Geometry check sheet. Reference: the model listing, model coordinates, mm. Round coordinates to 2 decimals unless told otherwise and drop trailing zeros. Order: outer loops, then holes, each group sorted by start corner. A loop starts at its lowest first (then second) coordinate and runs counter-clockwise, first axis right, second up. Notation, with made-up numbers: (-27.5, 39.25) - (16.5, 39.25) arc R9 ccw to (16.5, 43.25) - close; hole circle Ø8 at (86, 4). An arc over 180 degrees is marked (long way). Return JSON: item names as keys, results as strings. Group by question number.
Q1. Sectioned sample at C-C, the plane z = -10.5. Record the cut outline in (x, y).
Q2. Sectioned sample at A-A, the plane x = 5. Record the cut outline in (y, z).
Q3. Sectioned sample at D-D, the plane z = -18. Record the cut outline in (x, y).
Q4. Sectioned sample at B-B, the plane z = 0. Record the cut outline in (x, y).
Q5. Material ranges on line 1 along X through (y, z) = (1.5, 0); line 2 along X through (y, z) = (2.1, -2); line 3 along Z through (x, y) = (34, 2.3), recorded low to high.
Q6. Gauge pin test, flat ends, axial feed: pin 1 Ø3.5 at (x, z) = (0.52, -4.74) entering from -Y; pin 2 Ø1.5 at (y, z) = (2, -8.5) entering from +X; pin 3 Ø1.5 at (x, y) = (29.5, 1) entering from -Z; pin 4 Ø1.5 at (x, y) = (42, 2) entering from +Z. Record the tip position at first contact, or that the pin passes through.
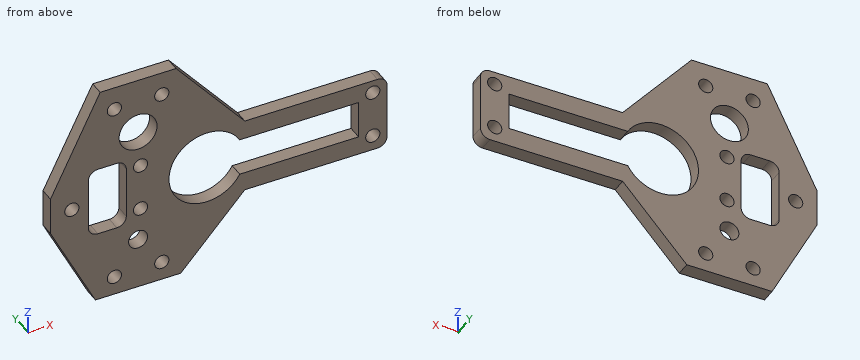
```python
from build123d import *

# Parameters (mm, degrees)
BASE_FLANGE1_DEPTH = 3
CUT_EXTRUDE1_REACH = 60.356
CUT_EXTRUDE2_REACH = 60.356
SKETCH3_R          = 1.5
SKETCH3_W          = 8
SKETCH3_H          = 15
CUT_EXTRUDE3_REACH = 60.356
SKETCH4_R          = 1.5
CUT_EXTRUDE4_REACH = 60.356
SKETCH5_R          = 2
SKETCH5_R_2        = 4
FILLET1_R          = 2


# Sheet-metal steps are written as plain solids
with BuildPart() as part:
    # Sketch1 → Base-Flange1 (new body)
    with BuildSketch(Plane(origin=(0, 0, 0), x_dir=(1, 0, 0), z_dir=(0, 1, 0))):
        Polygon((-18.480295105, -4), (-18.480295105, 4), (-9, 22.738303144), (9, 22.738303144), (22.519704895, 8), (52.519704895, 8), (52.519704895, -8), (22.519704895, -8), (8, -25.261696856), (-8, -25.261696856), align=None)
    extrude(amount=BASE_FLANGE1_DEPTH)

    # Sketch2 → Cut-Extrude1 (cut, up to next)
    with BuildSketch(Plane(origin=(0, 3, 0), x_dir=(1, 0, 0), z_dir=(0, 1, 0)), mode=Mode.PRIVATE) as cut_extrude1_sk1:
        with BuildLine():
            Line((21.447908125, 4), (46.519704895, 4))
            Line((46.519704895, 4), (46.519704895, -4))
            Line((46.519704895, -4), (21.447908125, -4))
            ThreePointArc((21.447908125, -4), (6.519704895, 0), (21.447908125, 4))
        make_face()
    cut_extrude1_tool1 = extrude(cut_extrude1_sk1.sketch, amount=-CUT_EXTRUDE1_REACH, mode=Mode.PRIVATE) & part.part
    add(cut_extrude1_tool1.solids().sort_by_distance((24.274518, 3, 0))[0], mode=Mode.SUBTRACT)

    # Sketch3 → Cut-Extrude2 (cut, up to next)
    with BuildSketch(Plane(origin=(0, 3, 0), x_dir=(1, 0, 0), z_dir=(0, 1, 0)), mode=Mode.PRIVATE) as cut_extrude2_sk1:
        with Locations(Location((-13.980295105, 0, 0), (0, 0, 270))):
            Circle(SKETCH3_R)
    cut_extrude2_tool1 = extrude(cut_extrude2_sk1.sketch, amount=-CUT_EXTRUDE2_REACH, mode=Mode.PRIVATE) & part.part
    # Sketch3 → Cut-Extrude2 (cut, up to next)
    with BuildSketch(Plane(origin=(0, 3, 0), x_dir=(1, 0, 0), z_dir=(0, 1, 0)), mode=Mode.PRIVATE) as cut_extrude2_sk2:
        with Locations((-6.480295105, 0)):
            Rectangle(SKETCH3_W, SKETCH3_H)
    cut_extrude2_tool2 = extrude(cut_extrude2_sk2.sketch, amount=-CUT_EXTRUDE2_REACH, mode=Mode.PRIVATE) & part.part
    add(cut_extrude2_tool1.solids().sort_by_distance((-13.980295, 3, 0))[0], mode=Mode.SUBTRACT)
    add(cut_extrude2_tool2.solids().sort_by_distance((-6.480295, 3, 0))[0], mode=Mode.SUBTRACT)

    # Sketch4 → Cut-Extrude3 (cut, up to next)
    with BuildSketch(Plane(origin=(0, 3, 0), x_dir=(1, 0, 0), z_dir=(0, 1, 0)), mode=Mode.PRIVATE) as cut_extrude3_sk1:
        with Locations(Location((-5, 18.738303144, 0), (0, 0, 270))):
            Circle(SKETCH4_R)
    cut_extrude3_tool1 = extrude(cut_extrude3_sk1.sketch, amount=-CUT_EXTRUDE3_REACH, mode=Mode.PRIVATE) & part.part
    # Sketch4 → Cut-Extrude3 (cut, up to next)
    with BuildSketch(Plane(origin=(0, 3, 0), x_dir=(1, 0, 0), z_dir=(0, 1, 0)), mode=Mode.PRIVATE) as cut_extrude3_sk2:
        with Locations(Location((5, 18.738303144, 0), (0, 0, 270))):
            Circle(SKETCH4_R)
    cut_extrude3_tool2 = extrude(cut_extrude3_sk2.sketch, amount=-CUT_EXTRUDE3_REACH, mode=Mode.PRIVATE) & part.part
    # Sketch4 → Cut-Extrude3 (cut, up to next)
    with BuildSketch(Plane(origin=(0, 3, 0), x_dir=(1, 0, 0), z_dir=(0, 1, 0)), mode=Mode.PRIVATE) as cut_extrude3_sk3:
        with Locations(Location((0.519704895, 4.738303144, 0), (0, 0, 270))):
            Circle(SKETCH4_R)
    cut_extrude3_tool3 = extrude(cut_extrude3_sk3.sketch, amount=-CUT_EXTRUDE3_REACH, mode=Mode.PRIVATE) & part.part
    # Sketch4 → Cut-Extrude3 (cut, up to next)
    with BuildSketch(Plane(origin=(0, 3, 0), x_dir=(1, 0, 0), z_dir=(0, 1, 0)), mode=Mode.PRIVATE) as cut_extrude3_sk4:
        with Locations(Location((-5, -20.261696856, 0), (0, 0, 270))):
            Circle(SKETCH4_R)
    cut_extrude3_tool4 = extrude(cut_extrude3_sk4.sketch, amount=-CUT_EXTRUDE3_REACH, mode=Mode.PRIVATE) & part.part
    # Sketch4 → Cut-Extrude3 (cut, up to next)
    with BuildSketch(Plane(origin=(0, 3, 0), x_dir=(1, 0, 0), z_dir=(0, 1, 0)), mode=Mode.PRIVATE) as cut_extrude3_sk5:
        with Locations(Location((5, -20.261696856, 0), (0, 0, 270))):
            Circle(SKETCH4_R)
    cut_extrude3_tool5 = extrude(cut_extrude3_sk5.sketch, amount=-CUT_EXTRUDE3_REACH, mode=Mode.PRIVATE) & part.part
    # Sketch4 → Cut-Extrude3 (cut, up to next)
    with BuildSketch(Plane(origin=(0, 3, 0), x_dir=(1, 0, 0), z_dir=(0, 1, 0)), mode=Mode.PRIVATE) as cut_extrude3_sk6:
        with Locations(Location((0.519704895, -5.261696856, 0), (0, 0, 270))):
            Circle(SKETCH4_R)
    cut_extrude3_tool6 = extrude(cut_extrude3_sk6.sketch, amount=-CUT_EXTRUDE3_REACH, mode=Mode.PRIVATE) & part.part
    # Sketch4 → Cut-Extrude3 (cut, up to next)
    with BuildSketch(Plane(origin=(0, 3, 0), x_dir=(1, 0, 0), z_dir=(0, 1, 0)), mode=Mode.PRIVATE) as cut_extrude3_sk7:
        with Locations(Location((49.519704895, 4.738303144, 0), (0, 0, 270))):
            Circle(SKETCH4_R)
    cut_extrude3_tool7 = extrude(cut_extrude3_sk7.sketch, amount=-CUT_EXTRUDE3_REACH, mode=Mode.PRIVATE) & part.part
    # Sketch4 → Cut-Extrude3 (cut, up to next)
    with BuildSketch(Plane(origin=(0, 3, 0), x_dir=(1, 0, 0), z_dir=(0, 1, 0)), mode=Mode.PRIVATE) as cut_extrude3_sk8:
        with Locations(Location((49.519704895, -5.261696856, 0), (0, 0, 270))):
            Circle(SKETCH4_R)
    cut_extrude3_tool8 = extrude(cut_extrude3_sk8.sketch, amount=-CUT_EXTRUDE3_REACH, mode=Mode.PRIVATE) & part.part
    add(cut_extrude3_tool1.solids().sort_by_distance((-5, 3, -18.738303))[0], mode=Mode.SUBTRACT)
    add(cut_extrude3_tool2.solids().sort_by_distance((5, 3, -18.738303))[0], mode=Mode.SUBTRACT)
    add(cut_extrude3_tool3.solids().sort_by_distance((0.519705, 3, -4.738303))[0], mode=Mode.SUBTRACT)
    add(cut_extrude3_tool4.solids().sort_by_distance((-5, 3, 20.261697))[0], mode=Mode.SUBTRACT)
    add(cut_extrude3_tool5.solids().sort_by_distance((5, 3, 20.261697))[0], mode=Mode.SUBTRACT)
    add(cut_extrude3_tool6.solids().sort_by_distance((0.519705, 3, 5.261697))[0], mode=Mode.SUBTRACT)
    add(cut_extrude3_tool7.solids().sort_by_distance((49.519705, 3, -4.738303))[0], mode=Mode.SUBTRACT)
    add(cut_extrude3_tool8.solids().sort_by_distance((49.519705, 3, 5.261697))[0], mode=Mode.SUBTRACT)

    # Sketch5 → Cut-Extrude4 (cut, up to next)
    with BuildSketch(Plane(origin=(0, 3, 0), x_dir=(1, 0, 0), z_dir=(0, 1, 0)), mode=Mode.PRIVATE) as cut_extrude4_sk1:
        with Locations(Location((0, 11.738303144, 0), (0, 0, 270))):
            Circle(SKETCH5_R)
    cut_extrude4_tool1 = extrude(cut_extrude4_sk1.sketch, amount=-CUT_EXTRUDE4_REACH, mode=Mode.PRIVATE) & part.part
    # Sketch5 → Cut-Extrude4 (cut, up to next)
    with BuildSketch(Plane(origin=(0, 3, 0), x_dir=(1, 0, 0), z_dir=(0, 1, 0)), mode=Mode.PRIVATE) as cut_extrude4_sk2:
        with Locations(Location((0, -13.261696856, 0), (0, 0, 270))):
            Circle(SKETCH5_R_2)
    cut_extrude4_tool2 = extrude(cut_extrude4_sk2.sketch, amount=-CUT_EXTRUDE4_REACH, mode=Mode.PRIVATE) & part.part
    add(cut_extrude4_tool1.solids().sort_by_distance((0, 3, -11.738303))[0], mode=Mode.SUBTRACT)
    add(cut_extrude4_tool2.solids().sort_by_distance((0, 3, 13.261697))[0], mode=Mode.SUBTRACT)

    # Fillet1
    fillet1_edges = [part.edges().sort_by_distance(p)[0] for p in [
        (52.519704895, 1.5, -8),
        (52.519704895, 1.5, 8),
        (-2.480295105, 1.5, -7.5),
        (-2.480295105, 1.5, 7.5),
        (-10.480295105, 1.5, 7.5),
        (-10.480295105, 1.5, -7.5),
    ]]
    fillet(fillet1_edges, radius=FILLET1_R)


solid = part.part
```
Reply:
{
 "1": {"outline": "(-15.19, 0) - (-1.57, 0) - (-1.57, 3) - (-15.19, 3) - close; (1.57, 0) - (20.23, 0) - (20.23, 3) - (1.57, 3) - close"},
 "2": {"outline": "(0, -22.74) - (3, -22.74) - (3, -20.24) - (0, -20.24) - close; (0, -17.24) - (3, -17.24) - (3, 18.76) - (0, 18.76) - close; (0, 21.76) - (3, 21.76) - (3, 25.26) - (0, 25.26) - close"},
 "3": {"outline": "(-11.4, 0) - (-6.31, 0) - (-6.31, 3) - (-11.4, 3) - close; (-3.69, 0) - (3.69, 0) - (3.69, 3) - (-3.69, 3) - close; (6.31, 0) - (13.35, 0) - (13.35, 3) - (6.31, 3) - close"},
 "4": {"outline": "(-18.48, 0) - (-15.48, 0) - (-15.48, 3) - (-18.48, 3) - close; (-12.48, 0) - (-10.48, 0) - (-10.48, 3) - (-12.48, 3) - close; (-2.48, 0) - (6.52, 0) - (6.52, 3) - (-2.48, 3) - close; (46.52, 0) - (52.52, 0) - (52.52, 3) - (46.52, 3) - close"},
 "5": {"line 1": "-18.48 to -15.48, -12.48 to -10.48, -2.48 to 6.52, 46.52 to 52.52", "line 2": "-18.48 to -10.48, -2.48 to 6.77, 46.52 to 52.52", "line 3": "-8 to -4, 4 to 8"},
 "6": {"pin 1": "y = 0", "pin 2": "x = 51.49", "pin 3": "z = -8", "pin 4": "z = 8"}
}
